Solid Edge part; units mm, degrees
sketch "Sketch1" plane through (0, 0, 0) normal (0, -1, 0) x (1, 0, 0)
  line L0 (0, -8) -> (1, -8)
  line L1 (1, -8) -> (1, -0.501)
  line L2 (1, -0.501) -> (0.87, -0.101)
  line L3 (0.87, -0.101) -> (0.87, 0)
  line L4 (0.87, 0) -> (2, 0)
  line L5 (2, 0) -> (1.8863, 1.3)
  line L6 (1.8863, 1.3) -> (0, 1.3)
  dimension "D1" = 0.87
  dimension "D2" = 1
  dimension "D3" = 1.8863
revolve "RevolvedProtrusion1" add sketch "Sketch1" angle 360 about axis through (0, 0, 6) along (0, 0, -1)
fillet "Round_1" radius 0.6 1 edges at (-1.8863, 0, 1.3)
sketch "Sketch2" plane through (0, 0, 0) normal (0, -1, 0) x (1, 0, 0)
  line L0 (-0.25, 1.3) -> (-0.25, 0.8)
  line L1 (-0.25, 0.8) -> (0.25, 0.8)
  line L2 (0.25, 0.8) -> (0.25, 1.3)
  line L3 (0.25, 1.3) -> (-0.25, 1.3)
  dimension "D1" = 0.25
  dimension "D2" = 0.25
extrude "ExtrudedCutout_1" cut sketch "Sketch2" along normal mid plane 4
cosmetic_thread "Thread_1" thread depth 7.499
fillet "Round_2" radius 0.1 1 edges at (-0.87, 0, 0)
chamfer "Chamfer_1" distance 0.0012 angle 30 1 edges at (-1, 0, -8) measured on face at (0.6867, 0.6467, -8)
properties material "Steel"
Source: CAD feature listing. Evaluate the final solid. Frame: model axes, mm. A direction names the side the tool comes from. Coordinates: 2 decimals unless noted, no trailing zeros. Loops run counter-clockwise (first coordinate to the right, second up) from the corner with the lowest first, then second, coordinate; pieces in that order, holes last. Notation, with made-up numbers: (45.5, 32) -> (89.5, 32) arc R9 cw to (89.5, 47) -> close; hole circle Ø1 at (-34, -23). An arc over 180 degrees is marked (long way). Answer in a Markdown table with one row per item. Add a question column.
Q1. Reachability of faces 1 (the face through (0, -1, -4)), 2 (the face through (1, 0, 1.3)) from +Z, -Z, +X, -X, +Y, -Y: full face, straight path, thin tool, end or side. Return the list, or none.
Q2. Ray query, line 1 along Z through (x, y) = (-1, -0.4); line 2 along X through (y, z) = (0.25, -7); line 3 along Z through (x, y) = (0, 0.2). Return the intervals inside material, ascending.
Q3. Section C-C on z = -6.25. Return the cut outline in (x, y).
Q4. Section D-D on z = 0.5. Return the cut outline in (x, y).
Q5. Contact query for flat-ended pins moving along their axis: pin 1 Ø2 at (x, z) = (0.5, -3.5) entering from +Y; pin 2 Ø0.6 at (y, z) = (0, 1) entering from -X; pin 3 Ø1.5 at (y, z) = (0.5, -5.5) entering from +X. Output: stop coordinate, or through.
Computed values:
| question | item | result |
|---|---|---|
| 1 | face 1 | -Z |
| 1 | face 2 | +Z, +X, -X, +Y, -Y |
| 2 | line 1 | z = 0 to 1.3 |
| 2 | line 2 | x = -0.97 to 0.97 |
| 2 | line 3 | z = -8 to 0.8 |
| 3 | outline | circle Ø2 at (0, 0) |
| 4 | outline | circle Ø3.91 at (0, 0) |
| 5 | pin 1 | stops at y = 1 |
| 5 | pin 2 | stops at x = -1.94 |
| 5 | pin 3 | stops at x = 1 |
